from build123d import *

# Parameters (mm, degrees)
SKETCH1_W           = 38.1
SKETCH1_H           = 38.1
BOSS_EXTRUDE1_DEPTH = 137.922
SKETCH2_W           = 34.925
SKETCH2_H           = 34.925
CUT_EXTRUDE1_DEPTH  = 138.922
CUT_EXTRUDE2_DEPTH  = 39.1


with BuildPart() as part:
    # Sketch1 → Boss-Extrude1 (new body)
    with BuildSketch(Plane.XY):
        with Locations((19.05, 19.05)):
            Rectangle(SKETCH1_W, SKETCH1_H)
    extrude(amount=BOSS_EXTRUDE1_DEPTH)

    # Sketch2 → Cut-Extrude1 (cut, through all)
    with BuildSketch(Plane.XY.offset(137.922)):
        with Locations((20.6375, 20.6375)):
            Rectangle(SKETCH2_W, SKETCH2_H)
    extrude(amount=-CUT_EXTRUDE1_DEPTH, mode=Mode.SUBTRACT)

    # Sketch3 → Cut-Extrude2 (cut, through all)
    with BuildSketch(Plane.XZ):
        Polygon((0, 137.922), (38.1, 137.922), (38.1, 115.924954744), align=None)
        Polygon((38.1, 0), (0, 0), (0, 21.997045256), align=None)
    extrude(amount=-CUT_EXTRUDE2_DEPTH, mode=Mode.SUBTRACT)


solid = part.part
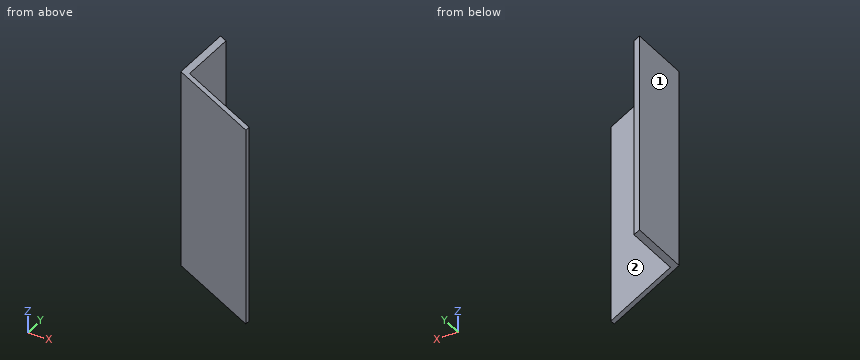
Verification items for the finished model (mm, model axes). Face numbers are marked on the shaded views. A direction names the side the tool comes from. Give positions to 0.01 mm unless a question says otherwise; leave off trailing zeros. Loops run counter-clockwise (first coordinate to the right, second up) from the corner with the lowest first, then second, coordinate; pieces in that order, holes last.
1) Depth check by flat-ended pin: pin 1 Ø12 at (x, z) = (23, 36.5) entering from +Y (3 decimals); pin 2 Ø4 at (y, z) = (20.5, 111.5) entering from +X (3 decimals); pin 3 Ø5 at (y, z) = (15.5, 17.5) entering from -X; pin 4 Ø5 at (x, y) = (5, 16.5) entering from +Z. Enter the tip coordinate at first touch or a pass-through.
2) Sectioned sample at C-C, the plane x = 23. Enter the section's corners in (y, z) (3 decimals), then the cut area to 3 significant figures.
3) Thickness scan on line 1 along Y through (x, z) = (26, 66.5) (3 decimals); line 2 along Z through (x, y) = (18, 2). Record the ranges inside material, lowest first.
4) Set-up check for the marked faces 1 and 2: record each of +Z, -Z, +X, -X, +Y, -Y from which the full face is reachable in a straight line by a thin tool's end or side.
5) Sectioned sample at A-A, the plane z = 24.5. Enter the section's corners in (x, y) (3 decimals).
6) Sectioned sample at B-B, the plane y = 16.5. Enter the section's corners in (x, z) (3 decimals), then the cut area to 3 significant figures.
Answers:
1. pin 1: stops at y = 3.175
1. pin 2: stops at x = 3.175
1. pin 3: passes through
1. pin 4: stops at z = 136.48
2. outline: (0, 8.718) - (3.175, 8.718) - (3.175, 124.643) - (0, 124.643) - close
2. area: 368 mm2
3. line 1: y = 0 to 3.175
3. line 2: z = 11.6 to 127.53
4. face 1: +Z, -Z, -X, +Y, -Y
4. face 2: +Z, -Z, +X, +Y
5. outline: (0, 0) - (38.1, 0) - (38.1, 3.175) - (3.175, 3.175) - (3.175, 38.1) - (0, 38.1) - close
6. outline: (0, 21.997) - (3.175, 20.164) - (3.175, 136.089) - (0, 137.922) - close
6. area: 368 mm2
